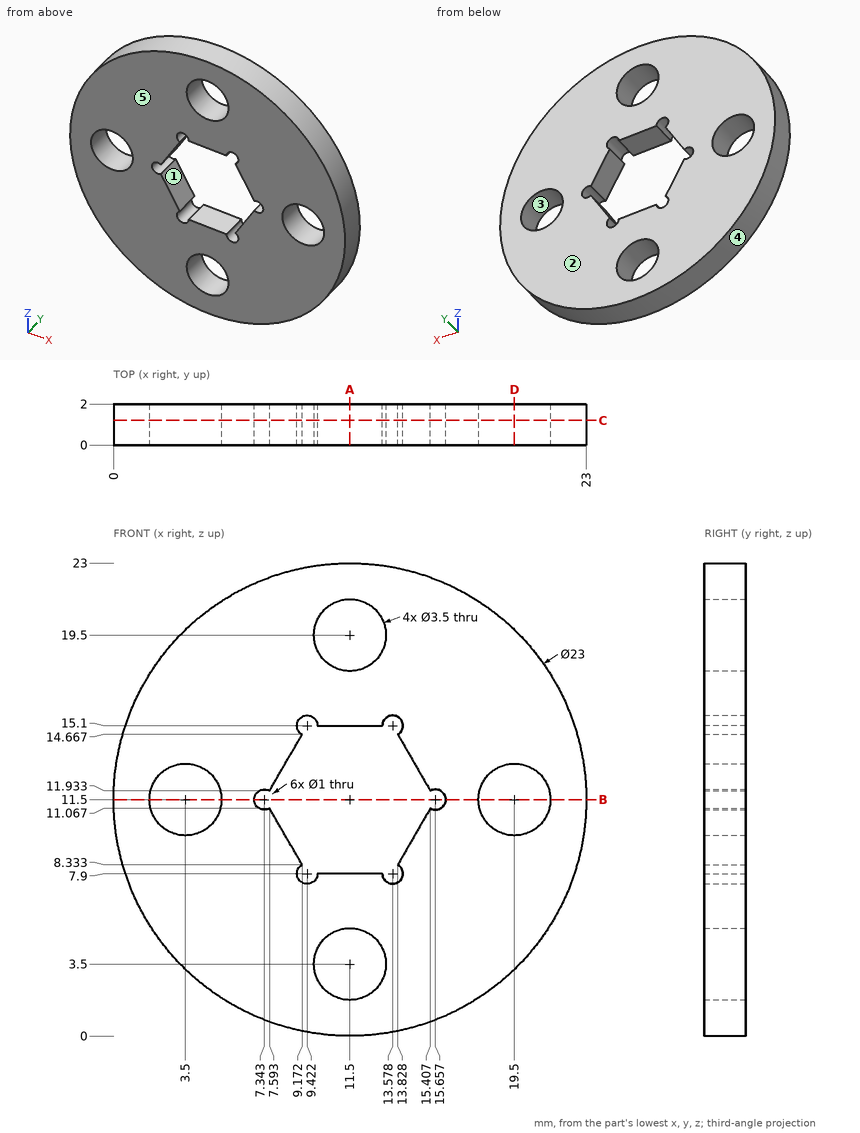
Print and shaded views of the part. All mm, measured from the part's lowest x, y and z. A direction names the side the tool comes from. Give positions to 0.01 mm unless a question says otherwise; leave off trailing zeros. Order: outer loops, then holes, each group sorted by start corner. A loop starts at its lowest first (then second) coordinate and runs counter-clockwise, first axis right, second up. Notation, with made-up numbers: M 0.25,25.5 L 44.25,25.5 A11 ccw 44.25,38.5 Z; hole C 81.25,0 d2. An arc over 180 degrees is marked long. Use one line per item in the form item = value.
Q1. Slice it at B-B, the plane z = 11.5. Write the cut outline in (x, y).
Conclusion:
outline = M 0,0 L 1.75,0 L 1.75,2 L 0,2 Z; M 5.25,0 L 6.84,0 L 6.84,2 L 5.25,2 Z; M 16.16,0 L 17.75,0 L 17.75,2 L 16.16,2 Z; M 21.25,0 L 23,0 L 23,2 L 21.25,2 Z
Q2. Slice it at A-A, the plane x = 11.5. Write the cut outline in (y, z).
Conclusion:
outline = M 0,0 L 2,0 L 2,1.75 L 0,1.75 Z; M 0,5.25 L 2,5.25 L 2,7.9 L 0,7.9 Z; M 0,15.1 L 2,15.1 L 2,17.75 L 0,17.75 Z; M 0,21.25 L 2,21.25 L 2,23 L 0,23 Z
Q3. Slice it at C-C, the plane y = 1.2. Write the cut outline in (x, z), and give its area (3 significant figures).
Conclusion:
outline = C 11.5,11.5 d23; hole C 3.5,11.5 d3.5; hole M 7.59,11.07 L 9.17,8.33 A0.5 ccw long 9.92,7.9 L 13.08,7.9 A0.5 ccw long 13.83,8.33 L 15.41,11.07 A0.5 ccw long 15.41,11.93 L 13.83,14.67 A0.5 ccw long 13.08,15.1 L 9.92,15.1 A0.5 ccw long 9.17,14.67 L 7.59,11.93 A0.5 ccw long Z; hole C 11.5,3.5 d3.5; hole C 11.5,19.5 d3.5; hole C 19.5,11.5 d3.5
area = 329 mm2
Q4. Wall check: probe 1 along X at (y, z) = (0.3, 11.75); probe 2 along X at (y, z) = (0.8, 11.5); probe 3 along Z at (x, y) = (12.75, 1.8) (1 decimal). Give the ranges that are in metal, low to high.
Conclusion:
probe_1 = 0 to 1.77, 5.23 to 6.91, 16.09 to 17.77, 21.23 to 23
probe_2 = 0 to 1.75, 5.25 to 6.84, 16.16 to 17.75, 21.25 to 23
probe_3 = 0.1 to 2.3, 4.7 to 7.9, 15.1 to 18.3, 20.7 to 22.9
Q5. Which spindle directions (+Z, -Z, +X, -X, +Y, -Y) get a long thin tool onto all of the face, cutting with end or side? Do the marked faces 1 and 2. Say none if no direction does.
Conclusion:
face_1 = +Y, -Y
face_2 = +Z, -Z, +X, -X, +Y
Q6. Pin check, flat tips, straight feed: P1, Ø1, axis at y = 0.5, z = 6.5, coming from the +X side; P2, Ø1, axis at y = 1.5, z = 17, coming from the +X side (1 decimal); P3, Ø1, axis at x = 15, y = 0.5, coming from the +Z side. Stop position of each tip, or through.
Conclusion:
P1 = 22.08
P2 = 21.9
P3 = 22.6
Q7. Pull direction X, two halves, no side cores. Call the marked faces 3, 4 and 5: released by +X, released by -X, zero draft, split by the parting line, or undercut.
Conclusion:
face_3 = undercut
face_4 = split by the parting line
face_5 = zero draft
Q8. Slice it at D-D, the plane x = 19.5. Write the cut outline in (y, z).
Conclusion:
outline = M 0,3.24 L 2,3.24 L 2,9.75 L 0,9.75 Z; M 0,13.25 L 2,13.25 L 2,19.76 L 0,19.76 Z
